Geometry check sheet. Reference: the model listing, model coordinates, mm. Face numbers are marked on the shaded views. A direction names the side the tool comes from. Give positions to 0.01 mm unless a question says otherwise; leave off trailing zeros. Loops run counter-clockwise (first coordinate to the right, second up) from the corner with the lowest first, then second, coordinate; pieces in that order, holes last. Notation, with made-up numbers: (33.5, 68.25) -> (37.5, 68.25) arc R12 ccw to (37.5, 83.25) -> close; hole circle Ø6 at (79.25, 89). An arc over 180 degrees is marked (long way). Answer in a Markdown table with one row per item. Add a question column.
Autodesk Inventor part; units mm, degrees
ref_plane "YZ Plane" through (0, 0, 0) normal (1, 0, 0) x (0, 1, 0)
ref_plane "XZ Plane" through (0, 0, 0) normal (0, 1, 0) x (-1, 0, 0)
ref_plane "XY Plane" through (0, 0, 0) normal (0, 0, 1) x (1, 0, 0)
sketch "Эскиз1" plane through (0, 0, 0) normal (0, 1, 0) x (-1, 0, 0)
  circle A0 centre (0, 0) radius 40
  dimension "d0" = 80
extrude "Выдавливание1" add sketch "Эскиз1" along normal blind 4
sketch "Эскиз2" plane through (0, 4, 0) normal (0, 1, 0) x (1, 0, 0)
  line L0 (-17, -10) -> (-27, -10)
  line L1 (-27, -10) -> (-27, 0)
  line L2 (-27, 0) -> (-17, 0)
  line L3 (-17, 0) -> (-17, -10)
  line L4 (27, -10) -> (17, -10)
  line L5 (17, -10) -> (17, 0)
  line L6 (17, 0) -> (27, 0)
  line L7 (27, 0) -> (27, -10)
  line L8 (5, -10) -> (-5, -10)
  line L9 (-5, -10) -> (-5, 0)
  line L10 (-5, 0) -> (5, 0)
  line L11 (5, 0) -> (5, -10)
  circle A0 centre (0, 0) radius 40
  line L12 (0, 40) -> (0, 16.8758)
  line L13 (40, 0) -> (27.344, 0)
  line L14 (0, 0) -> (0, 40)
  line L15 (40, 0) -> (0, 0)
  line L16 (39.6863, -5) -> (-39.6863, -5)
  dimension "d3" = 10
  dimension "d4" = 12
  dimension "d5" = 10
  dimension "d14" = 5
extrude "Выдавливание2" add sketch "Эскиз2" along normal blind 45 contours L0 L1 L16 L3 | L16 L1 L2 L3 | L16 L11 L8 L9 | L9 L10 L11 L16 | L16 L7 L4 L5 | L5 L6 L7 L16
sketch "Эскиз3" plane through (27, 4, 10) normal (1, 0, 0) x (0, 0, -1)
  line L0 (0, 45) -> (10, 45)
  line L1 (10, 0) -> (10, 45)
  circle A0 centre (5, 40) radius 2
  point P0 (10, -4)
  point P1 (5, 45)
  point P2 (10, 40)
  dimension "d8" = 5
  dimension "d9" = 4
  dimension "d20" = 0
extrude "Выдавливание3" cut sketch "Эскиз3" against normal blind 100
fillet "Сопряжение1" radius 5 6 edges at (-22, 49, 10) (-22, 49, 0) (0, 49, 10) (0, 49, 0) (22, 49, 10) (22, 49, 0)
sketch "Эскиз4" plane through (0, 4, 0) normal (0, 1, 0) x (1, 0, 0)
  line L0 (10, 25) -> (-10, 25)
  line L1 (-10, 25) -> (-10, 5)
  line L2 (-10, 5) -> (10, 5)
  line L3 (10, 5) -> (10, 25)
  circle A0 centre (0, 0) radius 40
  line L4 (0, 40) -> (0, 0)
  dimension "d15" = 20
  dimension "d16" = 20
  dimension "d17" = 5
extrude "Выдавливание4" cut sketch "Эскиз4" against normal blind 10 contours L3 L2 L4 L0 | L4 L2 L1 L0
sketch "Эскиз5" plane through (0, 4, 0) normal (0, 1, 0) x (1, 0, 0)
  line L0 (-27, -10) -> (-27, 0)
  line L1 (17, 0) -> (27, 0)
  line L2 (-27, -10) -> (27, -10)
  line L3 (27, -10) -> (27, 0)
  line L4 (27, 0) -> (-27, 0)
  line L5 (-27, 0) -> (-27, -10)
  point P0 (0, 0)
extrude "Выдавливание5" add sketch "Эскиз5" along normal blind 20
sketch "Эскиз6" plane through (0, 4, 0) normal (0, 1, 0) x (1, 0, 0)
  line L0 (-27, 0) -> (27, 0)
  line L1 (20, 0) -> (24, 0)
  line L2 (24, 0) -> (24, 20)
  line L3 (24, 20) -> (20, 20)
  line L4 (20, 20) -> (20, 0)
  line L5 (-24, 0) -> (-20, 0)
  line L6 (-20, 0) -> (-20, 20)
  line L7 (-20, 20) -> (-24, 20)
  line L8 (-24, 20) -> (-24, 0)
  line L9 (-5, -10) -> (5, -10)
  line L10 (-2, -10) -> (2, -10)
  line L11 (2, -10) -> (2, -30)
  line L12 (2, -30) -> (-2, -30)
  line L13 (-2, -30) -> (-2, -10)
  line L14 (-27, -10) -> (-17, -10)
  line L15 (-19, -10) -> (-15, -10)
  line L16 (-15, -10) -> (-15, -26)
  line L17 (-15, -26) -> (-19, -26)
  line L18 (-19, -26) -> (-19, -10)
  line L19 (27, -10) -> (-27, -10)
  line L20 (15, -10) -> (19, -10)
  line L21 (19, -10) -> (19, -26)
  line L22 (19, -26) -> (15, -26)
  line L23 (15, -26) -> (15, -10)
  line L24 (17, 0) -> (17, -10)
  line L25 (0, 0) -> (0, 4.7699)
  line L26 (-17, -10) -> (-17, 0)
  line L27 (-22, -10) -> (-22, 0)
  line L28 (17, -10) -> (27, -10)
  line L29 (22, -10) -> (22, 0)
  line L30 (-17, 0) -> (-27, 0)
  dimension "d23" = 4
  dimension "d24" = 20
  dimension "d25" = 16
  dimension "d26" = 20
  dimension "d27" = 0
extrude "Выдавливание6" add sketch "Эскиз6" along normal blind 15 contours L8 L7 L6 L0 | L14 L15 L16 L17 L18 | L4 L3 L2 L0 | L19 L21 L22 L23 | L9 L11 L12 L13
sketch "Эскиз7" plane through (27, 4, 10) normal (1, 0, 0) x (0, 0, -1)
  line L0 (-16, 0) -> (0, 0)
  line L1 (-16, 0) -> (0, 15)
  line L2 (0, 0) -> (0, 30)
  line L3 (10, 0) -> (10, 30)
  line L4 (30, 0) -> (30, 15)
  line L5 (10, 15) -> (30, 0)
  line L6 (50, 0) -> (-30, 0)
  line L7 (-30, 0) -> (50, 0)
  line L8 (50, 0) -> (50, -10)
  line L9 (50, -10) -> (-30, -10)
  line L10 (-30, -10) -> (-30, 0)
  arc A0 (10, 40) -> (0, 40) centre (5, 40) ccw
  line L11 (10, 0) -> (5, 0)
  line L12 (5, 0) -> (5, 45)
  line L13 (5, 45) -> (10, 45)
  line L14 (10, 45) -> (10, 0)
  line L15 (5, 45) -> (0, 45)
  line L16 (0, 45) -> (0, 0)
  line L17 (0, 0) -> (5, 0)
  line L18 (5, 0) -> (5, 45)
  point P0 (10, -4)
  dimension "d32" = 0
extrude "Выдавливание7" cut sketch "Эскиз7" against normal mid plane 1000 keep common part
sketch "Эскиз8" plane through (0, 4, 0) normal (0, 1, 0) x (1, 0, 0)
  circle A0 centre (0, 0) radius 36
  circle A1 centre (0, 0) radius 40
  circle A2 centre (0, 0) radius 32
  line L0 (-19, -10) -> (-15, -10)
  line L1 (-19, -10) -> (-15, -10)
  line L2 (-15, -10) -> (-15, -28.2666)
  line L3 (-15, -28.2666) -> (-19, -28.2666)
  line L4 (-19, -28.2666) -> (-19, -10)
  line L5 (19, -10) -> (19, -26)
  line L6 (19, -10) -> (15, -10)
  line L7 (15, -10) -> (15, -28.2666)
  line L8 (15, -28.2666) -> (19, -28.2666)
  line L9 (19, -28.2666) -> (19, -10)
  line L10 (-2, -26) -> (-2, -10)
  line L11 (-2, -10) -> (2, -10)
  line L12 (2, -10) -> (2, -36)
  line L13 (2, -36) -> (-2, -36)
  line L14 (-2, -36) -> (-2, -10)
  line L15 (20, 0) -> (20, 20)
  line L16 (20, 0) -> (24, 0)
  line L17 (24, 0) -> (24, 26.8328)
  line L18 (24, 26.8328) -> (20, 26.8328)
  line L19 (20, 26.8328) -> (20, 0)
  line L20 (-20, 0) -> (20, 0)
  line L21 (-20, 0) -> (-24, 0)
  line L22 (-24, 0) -> (-24, 26.8328)
  line L23 (-24, 26.8328) -> (-20, 26.8328)
  line L24 (-20, 26.8328) -> (-20, 0)
  point P0 (0, -40)
  point P1 (0, -36)
  point P2 (0, -32)
  point P3 (-20, 24.98)
  point P4 (-24, 21.166)
  point P5 (24, 21.166)
  point P6 (20, 24.98)
  point P7 (19, -25.7488)
  point P8 (-2, -31.9374)
  point P9 (2, -31.9374)
  point P10 (-19, -25.7488)
  dimension "d33" = 4
  dimension "d34" = 4
extrude "Выдавливание8" add sketch "Эскиз8" along normal blind 4 contours A0 L12 A2 L8 L9 L5 L17 | L18 L19 A2 L24 L23 A0 | L17 A2 L19 L18 | A0 L14 A2 L12 | L22 A2 L4 L3 L14 A0 | L23 L24 A2 L22 | L17 L16 L15 L19 A2 | A2 L14 L10 L11 L12 | A2 L24 L21 L22 | L7 L6 L5 A2 | A2 L5 L9 L8 | L4 L0 L2 A2 | A2 L3 L4
sketch "Эскиз9" plane through (0, 0, 0) normal (0, -1, 0) x (1, 0, 0)
  circle A0 centre (0, 0) radius 36
  circle A1 centre (0, 0) radius 32
extrude "Выдавливание9" add sketch "Эскиз9" along normal blind 4
sketch "Эскиз10" plane through (0, 0, 0) normal (0, -1, 0) x (1, 0, 0)
  line L0 (-18.9031, -19.8094) -> (-14.76, -19.8094)
  line L1 (-14.76, -19.8094) -> (-14.76, -11.0052)
  line L2 (-14.76, -11.0052) -> (-18.9031, -11.0052)
  line L3 (-18.9031, -11.0052) -> (-18.9031, -19.8094)
  point P0 (0, 0)
extrude "Выдавливание10" add sketch "Эскиз10" along normal blind 35
properties part number "типа подшипник"
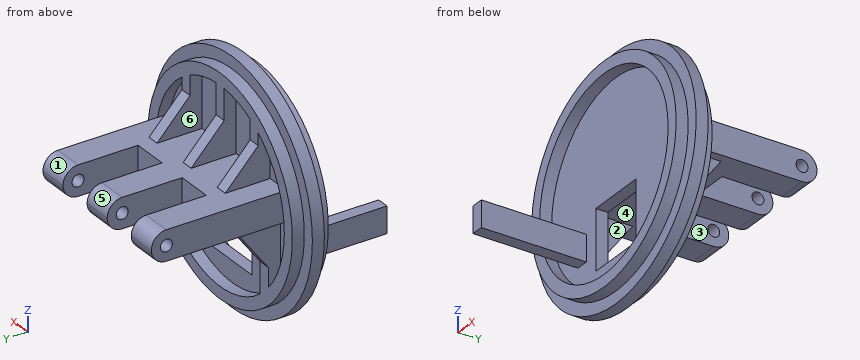
1. Sectioned sample at B-B (y = 2.5). Enter the section's corners in (x, z).
2. Material ranges on L1, parallel to X at y = 31.5, z = 3; L2, parallel to Y at x = -1, z = 5; L3, parallel to Z at x = 2, y = 41, recorded low to high. Write a range as from..to.
3. Gauge pin test, flat ends, axial feed: pin 1 Ø16.5 at (y, z) = (13, 17) entering from +X; pin 2 Ø4.5 at (y, z) = (15, 16) entering from +X; pin 3 Ø5 at (y, z) = (44, 5) entering from -X; pin 4 Ø24 at (x, z) = (-8, -7) entering from -Y. Record the tip position at first contact, or that the pin passes through.
4. Release check for a two-part mould opening along X. For the marked faces 4, 5 and 6 record: released by +X, released by -X, zero draft, split by the parting line, or undercut.
5. Sectioned sample at C-C (x = -13). Enter the section's corners in (y, z), plus the area to 3 significant figures.
6. Sectioned sample at D-D (y = -21). Enter the section's corners in (x, z), plus the area to 3 significant figures.
7. Sectioned sample at A-A (x = 0). Count the separate pieces of the cut face and the enclosed holes in it, plus the area to 3 significant figures.
8. Access from +Z, -Z, +X, -X, +Y, -Y to the whole of each face (thin tool, end or side, straight path). Record for the marked faces 1, 2 and 3.
Response:
| question | item | result |
|---|---|---|
| 1 | outline | circle Ø80 at (0, 0); hole (-10, -25) -> (10, -25) -> (10, -5) -> (-10, -5) -> close |
| 2 | L1 | x = -27..-17, -5..5, 17..27 |
| 2 | L2 | y = 0..42, 46..49 |
| 2 | L3 | z = 0..10 |
| 3 | pin 1 | stops at x = 34.45 |
| 3 | pin 2 | stops at x = 19 |
| 3 | pin 3 | stops at x = -27 |
| 3 | pin 4 | stops at y = -35 |
| 4 | face 4 | undercut |
| 4 | face 5 | zero draft |
| 4 | face 6 | undercut |
| 5 | outline | (-4, -33.57) -> (0, -33.57) -> (0, -37.83) -> (4, -37.83) -> (4, -33.57) -> (8, -33.57) -> (8, -29.24) -> (4, -29.24) -> (4, 0) -> (24, 0) -> (24, 10) -> (4, 10) -> (4, 29.24) -> (8, 29.24) -> (8, 33.57) -> (4, 33.57) -> (4, 37.83) -> (0, 37.83) -> (0, 33.57) -> (-4, 33.57) -> (-4, 29.24) -> (0, 29.24) -> (0, -29.24) -> (-4, -29.24) -> close |
| 5 | area | 572 mm2 |
| 6 | outline | (-18.9, -19.81) -> (-14.76, -19.81) -> (-14.76, -11.01) -> (-18.9, -11.01) -> close |
| 6 | area | 36.5 mm2 |
| 7 | separate pieces | 2 |
| 7 | enclosed holes | 1 |
| 7 | area | 883 mm2 |
| 8 | face 1 | +Z, +X, -X, +Y |
| 8 | face 2 | +Y |
| 8 | face 3 | +Z, -Z, +Y |
